```python
from build123d import *

# Parameters (mm, degrees)
BOSS_EXTRUDE1_DEPTH     = 57
SKETCH2_R               = 37.5
BOSS_EXTRUDE2_DEPTH     = 2
CUT_EXTRUDE1_DEPTH      = 210.155863705
CUT_EXTRUDE1_DEPTH_BACK = 210.155863705
SKETCH3_W               = 110
SKETCH3_H               = 54


with BuildPart() as part:
    # Sketch1 → Boss-Extrude1 (new, symmetric)
    with BuildSketch(Plane.XY):
        with BuildLine():
            Line((-165, -58.5), (-165, 58.5))
            Line((-165, 58.5), (0, 50))
            ThreePointArc((0, 50), (50, 0), (0, -50))
            Line((0, -50), (-165, -58.5))
        make_face()
    extrude(amount=BOSS_EXTRUDE1_DEPTH, both=True)

    # Sketch2 → Boss-Extrude2 (add)
    with BuildSketch(Plane.ZY.offset(165)):
        Circle(SKETCH2_R)
    extrude(amount=BOSS_EXTRUDE2_DEPTH)

    # Sketch3 → Cut-Extrude1 (cut, two sides: drawn at the far end of the back side and taken through both)
    with BuildSketch(Plane(origin=(2.568940095, 49.867660662, 0), x_dir=(0.9986757297720645, -0.05144693153371229, 0), z_dir=(0.051446931533712284, 0.9986757297720644, 0)).offset(-CUT_EXTRUDE1_DEPTH_BACK)):
        with Locations((-5, 0)):
            Rectangle(SKETCH3_W, SKETCH3_H)
    extrude(amount=CUT_EXTRUDE1_DEPTH + CUT_EXTRUDE1_DEPTH_BACK, mode=Mode.SUBTRACT)


solid = part.part
```
Can you work these out from the model? Positions are in its coordinate system, mm. A direction names the side the tool comes from. Give positions to 0.01 mm unless a question says otherwise; leave off trailing zeros. Loops run counter-clockwise (first coordinate to the right, second up) from the corner with the lowest first, then second, coordinate; pieces in that order, holes last. Notation, with made-up numbers: M 7,-13 L 42,-13 A14 ccw 42,-1 Z; hole C -11.5,61 d10. An arc over 180 degrees is marked long. One line per item, written item: value.
(1) Suppose I cut it at D-D on z = -18. List the corners of the cut face in (x, y) for me, plus the area to 3 significant figures.
Returned:
outline: M -167,-32.9 L -165,-32.9 L -165,-58.5 L -62.82,-53.24 L -57.35,52.95 L -165,58.5 L -165,32.9 L -167,32.9 Z
area: 11,800 mm^2
(2) We'd pull the mould along Z, two halves only. Please class faces 1 (the face through (-56, 1, -57)), 2 (the face through (-99.678, -55.135, 0.798)), 3 (the face through (-56, 1, 57)), 4 (the face through (-6, -4, -27)): released by +Z, released by -Z, zero draft, split by the parting line, or undercut.
Returned:
face 1: released by -Z
face 2: zero draft
face 3: released by +Z
face 4: undercut
(3) Suppose I cut it at B-B on y = 5. List the corners of the cut face in (x, z) for me.
Returned:
outline: M -167,-37.17 L -165,-37.17 L -165,-57 L 49.75,-57 L 49.75,-27 L -59.82,-27 L -59.82,27 L 49.75,27 L 49.75,57 L -165,57 L -165,37.17 L -167,37.17 Z
(4) Suppose I cut it at A-A on z = 0. List the corners of the cut face in (x, y) for me, plus the area to 3 significant figures.
Returned:
outline: M -167,-37.5 L -165,-37.5 L -165,-58.5 L -62.82,-53.24 L -57.35,52.95 L -165,58.5 L -165,37.5 L -167,37.5 Z
area: 11,900 mm^2
(5) Suppose I cut it at C-C on x = -82.5. List the corners of the cut face in (y, z) for me.
Returned:
outline: M -54.25,-57 L 54.25,-57 L 54.25,57 L -54.25,57 Z
(6) Which directions (+Z, -Z, +X, -X, +Y, -Y) give clear straight access to the entire face, cutting with the end or side of a thin tool? Please do faces 5 (the face through (-165.99, 37.18, -4.88)), 6 (the face through (49.988, 1.099, -41.79)), 7 (the face through (-60.125, -0.884, 0.378)).
Returned:
face 5: -X
face 6: +Z, -Z, +X
face 7: +X, -Y
(7) Will these pins go through, and if not, where does the flat tip stop? pin 1 (6 mm diameter, centred on y = -30, z = 19.5, fed in from +X); pin 2 (3 mm diameter, centred on x = 26, z = -45, fed in from -Y).
Returned:
pin 1: x = -61.47
pin 2: y = -43.59
(8) I need wall thicknesses on line 1 (Z direction, x = -20.5, y = -0.5); line 2 (X direction, y = 7.5, z = 24.5); line 3 (X direction, y = -15, z = 44). Which ranges of each line are inside material? Lowest first, please.
Returned:
line 1: -57 to -27, 27 to 57
line 2: -167 to -59.69
line 3: -165 to 47.7
